Could you check a few things on this model? Use its own coordinates, in mm. Face numbers are marked on the shaded views. A direction names the side the tool comes from. Coordinates: 2 decimals unless noted, no trailing zeros. Order: outer loops, then holes, each group sorted by start corner. A loop starts at its lowest first (then second) coordinate and runs counter-clockwise, first axis right, second up. Notation, with made-up numbers: (-14, -29.75) -> (13, -29.75) arc R35 ccw to (13, 5.25) -> close; hole circle Ø10 at (41.5, 60.25). An arc over 180 degrees is marked (long way). Return JSON: item names as keys, results as strings. Group by question number.
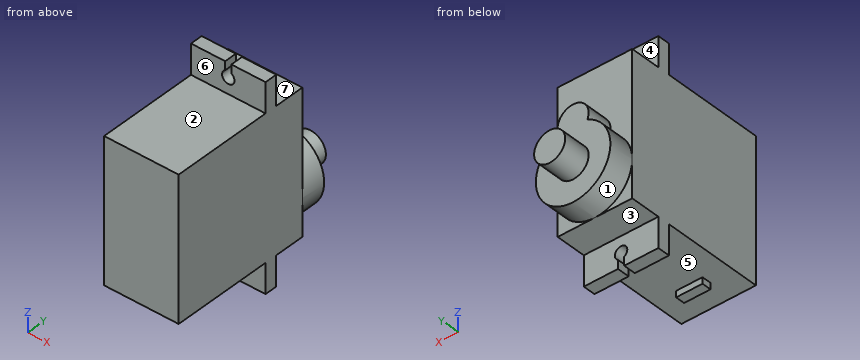
Autodesk Inventor part; units mm, degrees
ref_plane "YZ Plane" through (0, 0, 0) normal (1, 0, 0) x (0, 1, 0)
ref_plane "XZ Plane" through (0, 0, 0) normal (0, 1, 0) x (-1, 0, 0)
ref_plane "XY Plane" through (0, 0, 0) normal (0, 0, 1) x (1, 0, 0)
sketch "Sketch1" plane through (0, 0, 0) normal (0, 1, 0) x (-1, 0, 0)
  line L0 (-6, -6) -> (6, -6)
  line L1 (6, -6) -> (6, 16.9)
  line L2 (6, 16.9) -> (-6, 16.9)
  line L3 (-6, 16.9) -> (-6, -6)
  point P0 (0, 0)
  dimension "d0" = 12
  dimension "d1" = 22.9
extrude "Extrusion1" add sketch "Sketch1" along normal blind 16.3
sketch "Sketch2" plane through (0, 16.3, 0) normal (0, 1, 0) x (1, 0, 0)
  line L0 (6, 10.8) -> (6, -21.7)
  line L1 (-6, -21.7) -> (-6, 10.8)
  line L2 (6, 8.55) -> (6, -19.45)
  line L3 (-6, -19.45) -> (-6, 8.55)
  arc A0 (-0.5, 9.416) -> (0.5, 9.416) centre (0, 8.55) ccw
  line L4 (0.5, 10.8) -> (0.5, 9.416)
  line L5 (-0.5, 10.8) -> (-0.5, 9.416)
  line L6 (-6, 10.8) -> (-0.5, 10.8)
  line L7 (0.5, 10.8) -> (6, 10.8)
  arc A1 (0.5, -20.316) -> (-0.5, -20.316) centre (0, -19.45) ccw
  line L8 (-0.5, -21.7) -> (-0.5, -20.316)
  line L9 (0.5, -21.7) -> (0.5, -20.316)
  line L10 (6, -21.7) -> (0.5, -21.7)
  line L11 (-0.5, -21.7) -> (-6, -21.7)
  line L12 (-6, -16.9) -> (6, -16.9)
  line L13 (6, 6) -> (-6, 6)
  point P0 (0, 0)
  dimension "d5" = 32.5
  dimension "d12" = 28
  dimension "d28" = 27.7
  dimension "d29" = 22.9
  dimension "d32" = 2.55
  dimension "d33" = 4.8
  dimension "d34" = 1
  dimension "d35" = 12
extrude "Extrusion2" add sketch "Sketch2" along normal blind 2
sketch "Sketch3" plane through (0, 18.3, 0) normal (0, 1, 0) x (1, 0, 0)
  line L0 (-6, 6) -> (6, 6)
  line L1 (6, 6) -> (6, -16.9)
  line L2 (6, -16.9) -> (-6, -16.9)
  line L3 (-6, -16.9) -> (-6, 6)
  point P0 (0, 0)
  dimension "d9" = 22.9
extrude "Extrusion3" add sketch "Sketch3" along normal blind 4.9
sketch "Sketch4" plane through (0, 23.2, 0) normal (0, 1, 0) x (1, 0, 0)
  arc A0 (2.3077, -5.5385) -> (-2.3077, -5.5385) centre (0, 0) ccw
  arc A1 (-2.3077, -5.5385) -> (2.3077, -5.5385) centre (0, -6.5) ccw
extrude "Extrusion4" add sketch "Sketch4" along normal blind 4.1
sketch "Sketch5" plane through (0, 27.3, 0) normal (0, 1, 0) x (1, 0, 0)
  circle A0 centre (0, 0) radius 2.5
  dimension "d18" = 5
extrude "Extrusion5" add sketch "Sketch5" along normal blind 4.4
sketch "Sketch6" plane through (6, 0, -6) normal (0, 0, -1) x (-1, 0, 0)
  line L0 (0, 0) -> (0, 5.5)
  line L1 (0, 5.5) -> (12, 5.5)
  line L2 (6, 4) -> (8.125, 4)
  line L3 (3.875, 4) -> (8.125, 4)
  line L4 (8.125, 4) -> (8.125, 5.5)
  line L5 (8.125, 5.5) -> (3.875, 5.5)
  line L6 (3.875, 5.5) -> (3.875, 4)
  point P0 (6, 0)
  dimension "d22" = 5.5
  dimension "d23" = 4.25
extrude "Extrusion6" add sketch "Sketch6" along normal blind 1
sketch "Sketch7" plane through (0, 31.7, 0) normal (0, 1, 0) x (1, 0, 0)
  line L0 (-6, -16.9) -> (6, -16.9)
  line L1 (-6, 0) -> (-6, -16.9)
  point P0 (0, 0)
  dimension "d26" = 16.9
  dimension "d27" = 6
sketch "Sketch8" plane through (-6, 0, -6) normal (-1, 0, 0) x (0, 0, 1)
  line L0 (0, 0) -> (22.9, 0)
  line L1 (-4.8, 16.3) -> (0, 16.3)
  point P0 (6, 0)
  dimension "d30" = 16.3
properties part number "HD-1900A_Servo" material "ABS Plastic"
Q1. I need wall thicknesses on line 1 along X through (y, z) = (17.5, -8.55); line 2 along Z through (x, y) = (0, 17.6); line 3 along Y through (x, z) = (-2.5, -3.5). Which ranges of each line are inside material? Lowest first, please. Write a range as from..to.
Q2. I want a section at D-D on y = 8. Please give me the cut outline in (x, z), and give its area (3 significant figures).
Q3. We'd pull the mould along Y, two halves only. Please class the marked faces 5, 6 and 7: pulls with the +Y half, pulls with the -Y half, needs draft (parallel to the pull), parting line crosses it, or undercut.
Q4. I'm going to push flat-ended pins straight in: pin 1 Ø3 at (x, y) = (4.5, 22.5) entering from +Z; pin 2 Ø1.1 at (x, z) = (0, -6.5) entering from +Y; pin 3 Ø1.2 at (x, y) = (0.5, 5) entering from -Z; pin 4 Ø3 at (x, z) = (-2, -2.5) entering from +Y. Where does each tip first touch, or does it pass through?
Q5. On a 3-axis mill with a long thin cutter (end or side, diameter ignored), from which of +Z, -Z, +X, -X, +Y, -Y can I reach the whole of each face in a straight line? I mean the marked faces 1, 2, 3 and 4. Say none if no direction works.
Q6. I want a section at C-C on x = 4.5. Please give me the cut outline in (y, z), and give its area (3 significant figures).
Q7. I want a section at B-B on z = 6.5. Please give me the cut outline in (x, y), and give its area (3 significant figures).
Q8. I want a section at A-A on z = 19.45. Please give me the cut outline in (x, y).
Response values:
{
 "1": {"line 1": "x = -6..-1, 1..6", "line 2": "z = -7.55..18.45", "line 3": "y = 0..27.3"},
 "2": {"outline": "(-6, -6) -> (6, -6) -> (6, 16.9) -> (-6, 16.9) -> close", "area": "275 mm²"},
 "3": {"face 5": "undercut", "face 6": "pulls with the -Y half", "face 7": "needs draft"},
 "4": {"pin 1": "stops at z = 16.9", "pin 2": "stops at y = 27.3", "pin 3": "stops at z = -7", "pin 4": "stops at y = 31.7"},
 "5": {"face 1": "+Y", "face 2": "+Z, +X, -X, -Y", "face 3": "-Z, +X, -X, +Y", "face 4": "+Z, +X, -X, +Y"},
 "6": {"outline": "(0, -6) -> (16.3, -6) -> (16.3, -10.8) -> (18.3, -10.8) -> (18.3, -6) -> (23.2, -6) -> (23.2, -3.97) -> (27.3, -3.97) -> (27.3, 3.97) -> (23.2, 3.97) -> (23.2, 16.9) -> (18.3, 16.9) -> (18.3, 21.7) -> (16.3, 21.7) -> (16.3, 16.9) -> (0, 16.9) -> close", "area": "583 mm²"},
 "7": {"outline": "(-6, 0) -> (6, 0) -> (6, 23.2) -> (2.5, 23.2) -> (2.5, 27.3) -> (-2.5, 27.3) -> (-2.5, 23.2) -> (-6, 23.2) -> close", "area": "299 mm²"},
 "8": {"outline": "(-6, 16.3) -> (-1, 16.3) -> (-1, 18.3) -> (-6, 18.3) -> close; (1, 16.3) -> (6, 16.3) -> (6, 18.3) -> (1, 18.3) -> close"}
}
